The model under review builds one solid part; all positions refer to its coordinate system, in mm. Face numbers are marked on the shaded views. A direction names the side the tool comes from. Coordinates: 2 decimals unless noted, no trailing zeros. Order: outer loops, then holes, each group sorted by start corner. A loop starts at its lowest first (then second) coordinate and runs counter-clockwise, first axis right, second up. Notation, with made-up numbers: M 59.25,-24.75 L 68.25,-24.75 A26 ccw 68.25,-4.75 Z; hole C -30,-17 d8. An arc over 180 degrees is marked long. Answer in a Markdown table with one row per item.
from build123d import *

# Parameters (mm, degrees)
F1_DEPTH = 20
F2_R     = 8
F3_R     = 5
F4_R     = 2
F5_R     = 1.5
F6_DEPTH = 50
F7_R     = 1.5
F8_DEPTH = 82.9


with BuildPart() as f1:
    # F0 (on Top) → F1 (new body)
    with BuildSketch(Plane.XY):
        Polygon((33.438562, 71.225935), (28.438562, 71.225935), (28.438562, 63.225935), (23.438562, 63.225935), (23.438562, 29.225935), (28.438562, 29.225935), (28.438562, 21.225935), (33.438562, 21.225935), (33.438562, 29.225935), (38.438562, 29.225935), (38.438562, 63.225935), (33.438562, 63.225935), align=None)
    extrude(amount=F1_DEPTH)

    # F2
    f2_edges = [f1.edges().sort_by_distance(p)[0] for p in [
        (30.938562, 21.225935, 0),
        (30.938562, 71.225935, 0),
    ]]
    fillet(f2_edges, radius=F2_R)

    # F3
    f3_edges = [f1.edges().sort_by_distance(p)[0] for p in [
        (38.438562, 46.225935, 20),
        (23.438562, 46.225935, 20),
        (38.438562, 46.225935, 0),
        (23.438562, 46.225935, 0),
    ]]
    fillet(f3_edges, radius=F3_R)

    # F4
    f4_edges = [f1.edges().sort_by_distance(p)[0] for p in [
        (33.438562, 25.225935, 20),
        (33.438562, 67.225935, 20),
        (28.438562, 67.225935, 20),
        (28.438562, 25.225935, 20),
    ]]
    fillet(f4_edges, radius=F4_R)

    # F5 (on Right) → F6 (cut)
    with BuildSketch(Plane.YZ):
        with Locations((67.979599, 6.239843)):
            Circle(F5_R)
        with Locations((25.230938, 7.8)):
            Circle(F5_R)
    extrude(amount=F6_DEPTH, mode=Mode.SUBTRACT)

    # F7 (on Front) → F8 (cut)
    with BuildSketch(Plane.XZ):
        with Locations((30.938562, 17.55051)):
            Circle(F7_R)
        with Locations((30.933637, 2.5)):
            Circle(F7_R)
    extrude(amount=-F8_DEPTH, mode=Mode.SUBTRACT)


solid = f1.part
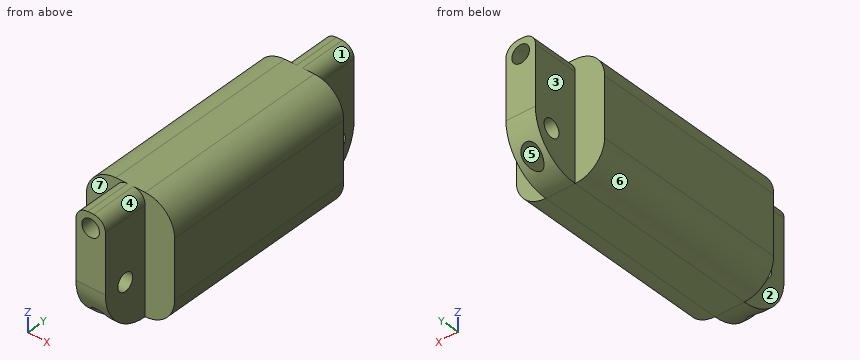
(1) The part is to be moulded in two halves that separate along X. For the marked faces 5, 6 and 7, say which applies: +X half, -X half, draft (parallel to the pull), parting line (faces both ways), or undercut.
Report:
| item | result |
|---|---|
| face 5 | undercut |
| face 6 | -X half |
| face 7 | draft |
(2) Take a section at C-C (y = 37). Write out the cut boundary in (x, z).
Report:
| item | result |
|---|---|
| outline | M 23.44,5 A5 ccw 28.44,0 L 33.44,0 A5 ccw 38.44,5 L 38.44,15 A5 ccw 33.44,20 L 28.44,20 A5 ccw 23.44,15 Z; hole C 30.93,2.5 d3; hole C 30.94,17.55 d3 |
(3) Take a section at D-D (x = 34.5). Write out the cut boundary in (y, z).
Report:
| item | result |
|---|---|
| outline | M 29.23,0.11 L 63.23,0.11 L 63.23,19.89 L 29.23,19.89 Z |
(4) Insertion check: P1, Ø4, axis at y = 68.5, z = 13.5, coming from the -X side; P2, Ø3.5, axis at x = 34, z = 6, coming from the +Y side; P3, Ø6.5, axis at y = 67.5, z = 9.5, coming from the +X side; P4, Ø2.5, axis at x = 30.94, z = 17.55, coming from the -Y side. Each pin has a flat end and moves straight along its axis. Give the tip position at first contact, or say it passes through.
Report:
| item | result |
|---|---|
| P1 | x = 28.44 |
| P2 | y = 71.22 |
| P3 | x = 33.44 |
| P4 | through |
(5) Take a section at B-B (z = 11.75). Write out the cut boundary in (x, y).
Report:
| item | result |
|---|---|
| outline | M 23.44,29.23 L 28.44,29.23 L 28.44,21.23 L 33.44,21.23 L 33.44,29.23 L 38.44,29.23 L 38.44,63.23 L 33.44,63.23 L 33.44,71.23 L 28.44,71.23 L 28.44,63.23 L 23.44,63.23 Z |
(6) To check wall thickness, follow line 1 (Z direction, x = 31.5, y = 49); line 2 (Y direction, x = 37.5, z = 16.5); line 3 (Y direction, x = 31.5, z = 7.8). State the ranges of each line that lie inside material, in increasing order. Write a range as [from, to].
Report:
| item | result |
|---|---|
| line 1 | [0, 1.11], [3.89, 16.16], [18.94, 20] |
| line 2 | [29.23, 63.23] |
| line 3 | [21.23, 23.73], [26.73, 71.22] |
(7) Machinability: for the marked faces 1, 2, 3 and 4, which of the approach directions +Z, -Z, +X, -X, +Y, -Y give a long, thin tool a straight path to every point of the face, cutting with its end or side? Answer none if there is none.
Report:
| item | result |
|---|---|
| face 1 | +Z, +X, +Y |
| face 2 | +Z, -Z, -X, -Y |
| face 3 | +Z, -Z, -X, +Y |
| face 4 | +Z, +X, -Y |
(8) Take a section at A-A (z = 3.5). Write out the cut boundary in (x, y).
Report:
| item | result |
|---|---|
| outline | M 23.67,29.23 L 28.44,29.23 L 28.44,22.61 L 29.82,22.61 L 29.82,69.84 L 28.44,69.84 L 28.44,63.23 L 23.67,63.23 Z; M 32.05,22.61 L 33.44,22.61 L 33.44,29.23 L 38.21,29.23 L 38.21,63.23 L 33.44,63.23 L 33.44,69.84 L 32.05,69.84 Z |
